from build123d import *
from build123d.topology import SkipClean

# Parameters (mm, degrees)
SKETCH1_R           = 5
SKETCH1_R_2         = 2.5
BOSS_EXTRUDE1_DEPTH = 5
SKETCH2_R           = 6.5
BOSS_EXTRUDE2_DEPTH = 2
CHAMFER1_SIZE       = 0.5
CUT_EXTRUDE1_DEPTH  = 0.5
CUT_EXTRUDE2_DEPTH  = 5


with BuildPart() as part:
    # Sketch1 → Boss-Extrude1 (new body)
    with BuildSketch(Plane.XY):
        Circle(SKETCH1_R)
        Circle(SKETCH1_R_2, mode=Mode.SUBTRACT)
    extrude(amount=-BOSS_EXTRUDE1_DEPTH)

    # Sketch2 → Boss-Extrude2 (add)
    with BuildSketch(Plane.XY):
        Circle(SKETCH2_R)
    extrude(amount=BOSS_EXTRUDE2_DEPTH)

    # Chamfer1
    chamfer1_edges = [part.edges().sort_by_distance(p)[0] for p in [
        (-6.5, 0, 2),
    ]]
    chamfer(chamfer1_edges, length=CHAMFER1_SIZE)

    # Sketch3 → Cut-Extrude1 (cut)
    with SkipClean():  # the faces are left unmerged after this step: merging them gives an invalid solid
        with BuildSketch(Plane(origin=(0, 0, 0), x_dir=(-1, 0, 0), z_dir=(0, 0, -1))):
            with BuildLine():
                Line((4.582575695, 2), (6.184658438, 2))
                ThreePointArc((6.184658438, 2), (6.5, 0), (6.184658438, -2))
                Line((6.184658438, -2), (4.582575695, -2))
                ThreePointArc((4.582575695, -2), (5, 0), (4.582575695, 2))
            make_face()
        extrude(amount=-CUT_EXTRUDE1_DEPTH, mode=Mode.SUBTRACT)

    # Sketch4 → Cut-Extrude2 (cut)
    with SkipClean():  # the faces are left unmerged after this step: merging them gives an invalid solid
        with BuildSketch(Plane(origin=(0, 0, -5), x_dir=(-1, 0, 0), z_dir=(0, 0, -1))):
            with BuildLine():
                Line((-1, 4.898979486), (-1, 3.872983346))
                ThreePointArc((-1, 3.872983346), (-2.828427125, 2.828427125), (-3.872983346, 1))
                Line((-3.872983346, 1), (-4.898979486, 1))
                ThreePointArc((-4.898979486, 1), (-3.535533906, 3.535533906), (-1, 4.898979486))
            make_face()
            with BuildLine():
                Line((1, 4.898979486), (1, 3.872983346))
                ThreePointArc((1, 3.872983346), (2.828427125, 2.828427125), (3.872983346, 1))
                Line((3.872983346, 1), (4.898979486, 1))
                ThreePointArc((4.898979486, 1), (3.535533906, 3.535533906), (1, 4.898979486))
            make_face()
            with BuildLine():
                Line((4.898979486, -1), (3.872983346, -1))
                ThreePointArc((3.872983346, -1), (2.828427125, -2.828427125), (1, -3.872983346))
                Line((1, -3.872983346), (1, -4.898979486))
                ThreePointArc((1, -4.898979486), (3.535533906, -3.535533906), (4.898979486, -1))
            make_face()
            with BuildLine():
                Line((-3.872983346, -1), (-4.898979486, -1))
                ThreePointArc((-4.898979486, -1), (-3.535533906, -3.535533906), (-1, -4.898979486))
                Line((-1, -4.898979486), (-1, -3.872983346))
                ThreePointArc((-1, -3.872983346), (-2.828427125, -2.828427125), (-3.872983346, -1))
            make_face()
        extrude(amount=-CUT_EXTRUDE2_DEPTH, mode=Mode.SUBTRACT)

    # Chamfer2: read off the stored shape, not the designer's step
    # Chamfer2 outline → Chamfer2 (revolve, cut)
    with SkipClean():  # the faces are left unmerged after this step: merging them gives an invalid solid
        with BuildSketch(Plane.XZ):
            Polygon((5, -4), (4, -5), (5, -5), align=None)
        revolve(axis=Axis((0, 0, 0), (0, 0, 1)), mode=Mode.SUBTRACT)


solid = part.part
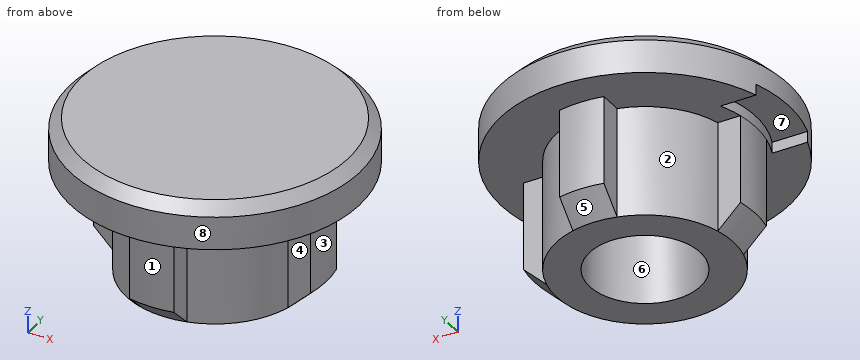
Source: CAD feature listing. Evaluate the final solid. Frame: model axes, mm. Face numbers are marked on the shaded views. A direction names the side the tool comes from. Give positions to 0.01 mm unless a question says otherwise; leave off trailing zeros. Write each loop counter-clockwise with the first axis right and the second up, starting at its lowest first coordinate (ties: lowest second). Pieces come first, ordered by that corner, then holes. Notation, with made-up numbers: M -14.75,-9 L 32.25,-9 A14 ccw 32.25,0 Z; hole C 75.5,55.25 d1. An arc over 180 degrees is marked long. Return JSON: item names as keys, results as strings. Group by question number.
1) First-contact query: pin 1 Ø1.5 at (x, y) = (0.5, 0.5) entering from -Z; pin 2 Ø6.5 at (x, y) = (-0.5, 1) entering from -Z; pin 3 Ø0.8 at (y, z) = (-4.5, -2.5) entering from -X; pin 4 Ø1.1 at (x, z) = (4.5, -3.5) entering from +Y. Flat tips, straight axial feed; report the tip coordinate or a pass-through.
2) Ray query, L1, parallel to Y at x = 0, z = -1.9; L2, parallel to Z at x = 0, y = 0.75; L3, parallel to X at y = 2.25, z = -1.5. Return the intervals inside material, ascending.
3) Cut plane B-B, the plane y = 0. Output: boundary loops of the cut face in (x, z), then the cut area to 3 significant figures.
4) Cut plane D-D, the plane z = 1. Output: boundary loops of the cut face in (x, y).
5) Cut plane A-A, the plane z = -3. Output: boundary loops of the cut face in (x, y).
6) Draft query along Y for the marked faces 5, 6, 7 and 8. Return one class per face: released by +Y, released by -Y, zero draft, split by the parting line, or undercut.
7) Set-up query: the marked faces 1, 2, 3 and 4. Return all of +Z, -Z, +X, -X, +Y, -Y with unobstructed straight access to the full face (end or side cutting, diameter ignored); none if empty.
8) Cut plane C-C, the plane x = 0. Output: boundary loops of the cut face in (y, z), then the cut area to 4 significant figures.
Data:
{
 "1": {"pin 1": "stops at z = 0", "pin 2": "stops at z = -5", "pin 3": "stops at x = -1", "pin 4": "stops at y = 1"},
 "2": {"L1": "y = -5 to -2.5, 2.5 to 5", "L2": "z = 0 to 2", "L3": "x = -3.31 to -1.09, 1.09 to 3.31"},
 "3": {"outline": "M -6.5,0.5 L -5,0.5 L -5,-4 L -4,-5 L -2.5,-5 L -2.5,0 L 2.5,0 L 2.5,-5 L 4,-5 L 5,-4 L 5,0 L 6.5,0 L 6.5,1.5 L 6,2 L -6,2 L -6.5,1.5 Z", "area": "49.0 mm²"},
 "4": {"outline": "C 0,0 d13"},
 "5": {"outline": "M -4.9,-1 L -3.87,-1 A4 ccw -1,-3.87 L -1,-4.9 A5 ccw 1,-4.9 L 1,-3.87 A4 ccw 3.87,-1 L 4.9,-1 A5 ccw 4.9,1 L 3.87,1 A4 ccw 1,3.87 L 1,4.9 A5 ccw -1,4.9 L -1,3.87 A4 ccw -3.87,1 L -4.9,1 A5 ccw Z; hole C 0,0 d5"},
 "6": {"face 5": "released by +Y", "face 6": "undercut", "face 7": "undercut", "face 8": "split by the parting line"},
 "7": {"face 1": "-Z, -Y", "face 2": "-Z, -X, +Y", "face 3": "-Z, +X", "face 4": "-Z, +X, -Y"},
 "8": {"outline": "M -6.5,0 L -5,0 L -5,-4 L -4,-5 L -2.5,-5 L -2.5,0 L 2.5,0 L 2.5,-5 L 4,-5 L 5,-4 L 5,0 L 6.5,0 L 6.5,1.5 L 6,2 L -6,2 L -6.5,1.5 Z", "area": "49.75 mm²"}
}
